```python
from build123d import *

# Parameters (mm, degrees)
SALIENTE_EXTRUIR1_DEPTH = 5
CROQUIS3_R              = 2
CORTAR_EXTRUIR1_DEPTH   = 10


with BuildPart() as part:
    # Croquis1 → Saliente-Extruir1 (new body)
    with BuildSketch(Plane(origin=(0, 0, 0), x_dir=(1, 0, 0), z_dir=(0, 1, 0))):
        with BuildLine():
            Line((391.11715601, -589.26903854), (409.134507606, -600.572222265))
            Line((409.134507606, -600.572222265), (431.070113816, -696.364244316))
            ThreePointArc((431.070113816, -696.364244316), (446.060284595, -707.511220058), (462.598816983, -716.196681165))
            Line((462.598816983, -716.196681165), (600.572192141, -684.601882766))
            ThreePointArc((600.572192141, -684.601882766), (611.492139331, -669.889063268), (620.044894414, -653.685277145))
            Line((620.044894414, -653.685277145), (588.295487999, -515.036734211))
            ThreePointArc((588.295487999, -515.036734211), (572.526223432, -503.540761802), (555.102156346, -494.752760164))
            Line((555.102156346, -494.752760164), (459.421279691, -516.662914968))
            Line((459.421279691, -516.662914968), (442.992177211, -506.356119167))
            ThreePointArc((442.992177211, -506.356119167), (408.224347097, -542.287830533), (391.11715601, -589.26903854))
        make_face()
    extrude(amount=SALIENTE_EXTRUIR1_DEPTH)

    # Croquis3 → Cortar-Extruir1 (cut)
    with BuildSketch(Plane.XZ):
        with Locations(Location((449.910379391, 702.169476818, 0), (0, 0, 270))):
            Circle(CROQUIS3_R)
        with Locations(Location((413.720365983, 545.892005433, 0), (0, 0, 270))):
            Circle(CROQUIS3_R)
        with Locations(Location((569.997837367, 509.701992025, 0), (0, 0, 270))):
            Circle(CROQUIS3_R)
        with Locations(Location((606.187850775, 665.97946341, 0), (0, 0, 270))):
            Circle(CROQUIS3_R)
    extrude(amount=-CORTAR_EXTRUIR1_DEPTH, mode=Mode.SUBTRACT)


solid = part.part
```
Design review of the part built by this model. Coordinates are the model's own, in mm. A direction names the side the tool comes from. Give positions to 0.01 mm unless a question says otherwise; leave off trailing zeros. Order: outer loops, then holes, each group sorted by start corner. A loop starts at its lowest first (then second) coordinate and runs counter-clockwise, first axis right, second up. Notation, with made-up numbers: (37.25, 52.25) -> (58.25, 52.25) arc R32 cw to (58.25, 90.25) -> close; hole circle Ø4 at (-3.5, 32). An arc over 180 degrees is marked (long way). Write item = value, one per line. Start each with the question number.
(1) To check wall thickness, follow line 1 along X through (y, z) = (3.9, 644); line 2 along Z through (x, y) = (485.5, 0.7); line 3 along X through (y, z) = (0.75, 581). State the ranges of each line that lie inside material, in increasing order.
(2) We need section C-C on x = 560. Write out the cut boundary in (y, z).
(3) We need section A-A on y = 1.4. Write out the cut boundary in (x, z).
(4) We need section B-B on z = 630. Write out the cut boundary in (x, y), plus the area to 3 significant figures.
(5) For pin 1 (1.5 mm diameter, centred on y = 3, z = 613, fed in from -X); pin 2 (1 mm diameter, centred on x = 549.5, y = 2.5, fed in from -Z); pin 3 (2 mm diameter, centred on x = 451.5, y = 0.5, fed in from -Z), all flat-tipped, find the tip position at first contact; note any pin that passes through.
(6) For faces 1 (the face through (507.931, 2.465, 505.554)), 2 (the face through (419.95, 2.46, 647.8)), list the 3-axis set-ups (+Z, -Z, +X, -X, +Y, -Y) from which the entire face can be reached by the end or side of a thin tool; tool diameter is ignored.
(7) Mouldability with a two-part tool opening along X and no side actions: class faces 3 (the face through (451.32, 2.46, 511.58)), 4 (the face through (445.84, 2.46, 707.37)), 5 (the face through (611.355, 2.465, 670.106)) as +X half, -X half, draft (parallel to the pull), parting line (faces both ways), or undercut.
Numbers:
q1.line_1 = 419.08 to 617.83
q1.line_2 = 510.69 to 710.95
q1.line_3 = 392.57 to 603.4
q2.outline = (0, 496.87) -> (5, 496.87) -> (5, 693.89) -> (0, 693.89) -> close
q3.outline = (391.12, 589.27) arc R120 ccw to (442.99, 506.36) -> (459.42, 516.66) -> (555.1, 494.75) arc R120 ccw to (588.3, 515.04) -> (620.04, 653.69) arc R120 ccw to (600.57, 684.6) -> (462.6, 716.2) arc R120 ccw to (431.07, 696.36) -> (409.13, 600.57) -> close; hole circle Ø4 at (413.72, 545.89); hole circle Ø4 at (449.91, 702.17); hole circle Ø4 at (570, 509.7); hole circle Ø4 at (606.19, 665.98)
q4.outline = (415.87, 0) -> (614.62, 0) -> (614.62, 5) -> (415.87, 5) -> close
q4.area = 994 mm^2
q5.pin_1 = 411.81
q5.pin_2 = 495.92
q5.pin_3 = 511.07
q6.face_1 = -Z, +Y, -Y
q6.face_2 = +Z, -X, +Y, -Y
q7.face_3 = undercut
q7.face_4 = -X half
q7.face_5 = +X half
